Verification items for the finished model (mm, model axes). Face numbers are marked on the shaded views. A direction names the side the tool comes from. Round coordinates to 2 decimals unless told otherwise and drop trailing zeros. Write each loop counter-clockwise with the first axis right and the second up, starting at its lowest first coordinate (ties: lowest second). Pieces come first, ordered by that corner, then holes. Notation, with made-up numbers: M -24,12 L 4,12 A5 cw 4,16 Z; hole C 64,-25.5 d7. An arc over 180 degrees is marked long. Write each question's results on one line, items separated by ' | '.
from build123d import *

# Parameters (mm, degrees)
SKETCH_2_R          = 45
SKETCH_2_R_2        = 22.5
EXTRUDE_1_DEPTH     = 5
EXTRUDE_2_DEPTH     = 10
FILLET_1_R          = 2
SKETCH_4_R          = 2
CUT_EXTRUDE_1_DEPTH = 88.183714076
SKETCH_5_R          = 27.5
SKETCH_5_R_2        = 22.5
EXTRUDE_3_DEPTH     = 5
SKETCH_6_R          = 0.85
CUT_EXTRUDE_2_DEPTH = 67.708320321


with BuildPart() as part:
    # 草图2 → 凸台-拉伸1 (new body)
    with BuildSketch(Plane(origin=(0, 0, 0), x_dir=(1, 0, 0), z_dir=(0, 1, 0))):
        with Locations(Location((0, 0, 0), (0, 0, 270))):
            Circle(SKETCH_2_R)
        with Locations(Location((0, 0, 0), (0, 0, 270))):
            Circle(SKETCH_2_R_2, mode=Mode.SUBTRACT)
    extrude(amount=EXTRUDE_1_DEPTH)

    # 草图3 → 凸台-拉伸2 (add)
    with BuildSketch(Plane.XZ):
        Polygon((-27, 25), (-27, -25), (-20, -25), (-20, -29), (-32, -29), (-32, -25), (-32, 25), (-32, 29), (-20, 29), (-20, 25), align=None)
        Polygon((20, -29), (20, -25), (27, -25), (27, 25), (20, 25), (20, 29), (32, 29), (32, 25), (32, -25), (32, -29), align=None)
    extrude(amount=EXTRUDE_2_DEPTH)

    # 圆角1
    fillet_1_edges = [part.edges().sort_by_distance(p)[0] for p in [
        (-32, -5, 29),
        (-32, -5, -29),
        (32, -5, -29),
        (32, -5, 29),
    ]]
    fillet(fillet_1_edges, radius=FILLET_1_R)

    # 草图4 → 切除-拉伸1 (cut, through all)
    with BuildSketch(Plane.XY.offset(29)):
        with Locations((-25, -5)):
            Circle(SKETCH_4_R)
        with Locations((25, -5)):
            Circle(SKETCH_4_R)
    extrude(amount=-CUT_EXTRUDE_1_DEPTH, mode=Mode.SUBTRACT)

    # 草图5 → 凸台-拉伸3 (add)
    with BuildSketch(Plane(origin=(0, 5, 0), x_dir=(1, 0, 0), z_dir=(0, 1, 0))):
        with Locations(Location((0, 0, 0), (0, 0, 270))):
            Circle(SKETCH_5_R)
        with Locations(Location((0, 0, 0), (0, 0, 270))):
            Circle(SKETCH_5_R_2, mode=Mode.SUBTRACT)
    extrude(amount=EXTRUDE_3_DEPTH)

    # 草图6 → 切除-拉伸2 (cut, through all)
    with BuildSketch(Plane(origin=(0, 10, 0), x_dir=(1, 0, 0), z_dir=(0, 1, 0))):
        with Locations(Location((0, 24.6, 0), (0, 0, 270))):
            Circle(SKETCH_6_R)
        with Locations(Location((24.6, 0, 0), (0, 0, 270))):
            Circle(SKETCH_6_R)
        with Locations(Location((0, -24.6, 0), (0, 0, 270))):
            Circle(SKETCH_6_R)
        with Locations(Location((-24.6, 0, 0), (0, 0, 270))):
            Circle(SKETCH_6_R)
    extrude(amount=-CUT_EXTRUDE_2_DEPTH, mode=Mode.SUBTRACT)


solid = part.part
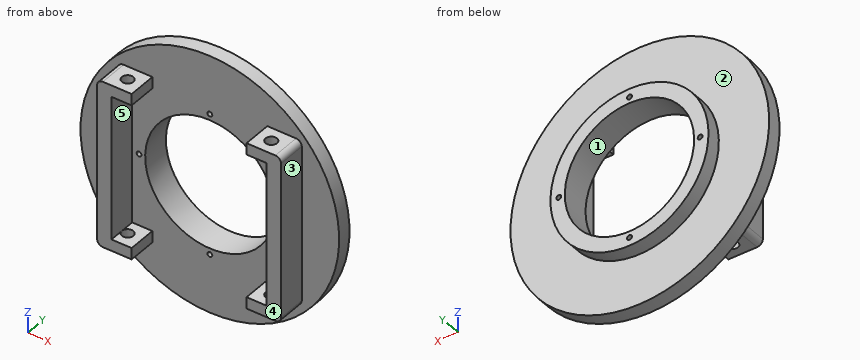
1) Sectioned sample at B-B, the plane z = 31.5. Record the cut outline in (x, y).
Calculated:
outline: M -32.14,0 L 32.14,0 L 32.14,5 L -32.14,5 Z
2) Sectioned sample at C-C, the plane z = -36.5. Record the cut outline in (x, y), and give its area (3 significant figures).
Calculated:
outline: M -26.32,0 L 26.32,0 L 26.32,5 L -26.32,5 Z | area: 263 mm²
3) Access from +Z, -Z, +X, -X, +Y, -Y to the whole of each face (thin tool, end or side, straight path). Record for the marked faces 4 and 5.
Calculated:
face 4: +Z, -Z, +X, -X, -Y | face 5: -Y
4) Sectioned sample at A-A, the plane x = 5. Record the cut outline in (y, z), and give its area (3 significant figures).
Calculated:
outline: M 0,-44.72 L 5,-44.72 L 5,-27.04 L 10,-27.04 L 10,-21.94 L 0,-21.94 Z; M 0,21.94 L 10,21.94 L 10,27.04 L 5,27.04 L 5,44.72 L 0,44.72 Z | area: 279 mm²
5) Material ranges on line 1 (X direction, y = -8, z = 3.5); line 2 (Y direction, x = -25, z = -26.9); line 3 (Z direction, x = 21.5, y = -1), recorded low to high. Write a range as [from, to].
Calculated:
line 1: x = [-32, -27], [27, 32] | line 2: y = [-10, -7], [-3, 5] | line 3: z = [-29, -25], [25, 29]
6) Draft check along X on the marked faces 1, 2 and 3. Enter one of: pulls with the +X half, pulls with the -X half, needs draft (parallel to the pull), parting line crosses it, or undercut.
Calculated:
face 1: undercut | face 2: needs draft | face 3: pulls with the +X half
7) Depth check by flat-ended pin: P1, Ø7.5, axis at x = 25, y = -4.5, coming from the +Z side; P2, Ø11, axis at y = -7, z = 11, coming from the -X side; P3, Ø3, axis at y = -3.5, z = 27.5, coming from the +X side; P4, Ø1.4, axis at x = 24.6, z = 0, coming from the +Y side. Enter the tip coordinate at first touch or a pass-through.
Calculated:
P1: stops at z = 29 | P2: stops at x = -32 | P3: stops at x = 32 | P4: passes through
